Verification items for this drawing (mm, ordinates from the low corner). A direction names the side the tool comes from. Round coordinates to 2 decimals unless told otherwise and drop trailing zeros. Write each loop counter-clockwise with the first axis right and the second up, starting at its lowest first coordinate (ties: lowest second). Pieces come first, ordered by that corner, then holes. Notation, with made-up numbers: (28, 6) -> (58, 6) arc R23 ccw to (58, 37) -> close; hole circle Ø3 at (45.5, -7.75). An arc over 180 degrees is marked (long way). Put each result on its own line as item: value. Start each with the question number.
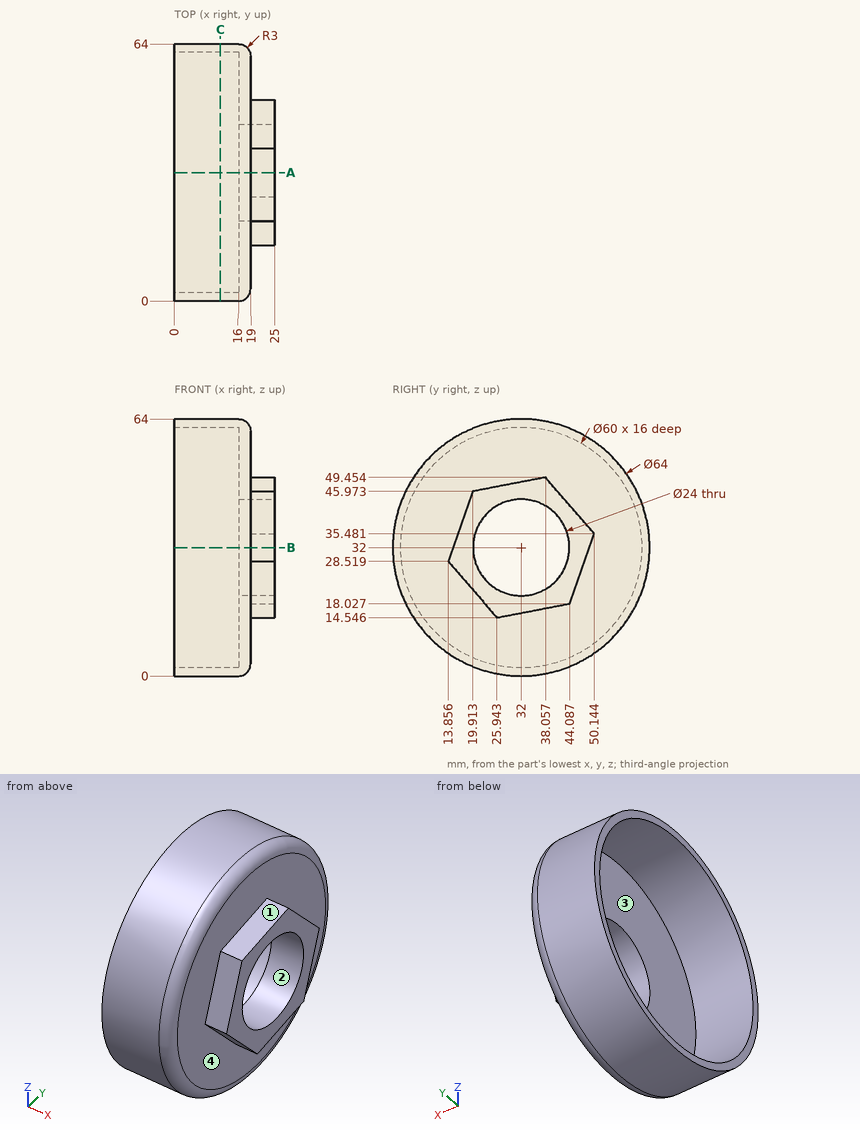
(1) Sectioned sample at B-B (z = 32). Record the cut outline in (x, y).
(2) Sectioned sample at C-C (x = 11.5). Record the cut outline in (y, z).
(3) Go/stop test with flat-tipped pins: pin 1 Ø1 at (y, z) = (39.5, 52.5) entering from +X; pin 2 Ø10 at (x, z) = (19.5, 51) entering from +Y (1 decimal); pin 3 Ø1 at (x, z) = (20.5, 53) entering from +Y (3 decimals); pin 4 Ø4 at (x, y) = (22.5, 14) entering from -Z. Record where each tip stops, or that it passes through.
(4) Material ranges on L1, parallel to Y at x = 7.25, z = 32; L2, parallel to Z at x = 2.75, y = 5 (1 decimal); L3, parallel to Z at x = 11.75, y = 34.5 (1 decimal), recorded low to high. Write a range as from..to.
(5) Sectioned sample at A-A (y = 32). Record the cut outline in (x, z).
(6) Set-up check for the marked faces 1, 2, 3 and 4: record each of +Z, -Z, +X, -X, +Y, -Y from which the full face is reachable in a straight line by a thin tool's end or side.
Found:
1. outline: (0, 0) -> (16, 0) arc R3 ccw to (19, 3) -> (19, 15.06) -> (25, 15.06) -> (25, 20) -> (16, 20) -> (16, 2) -> (0, 2) -> close; (0, 62) -> (16, 62) -> (16, 44) -> (25, 44) -> (25, 48.94) -> (19, 48.94) -> (19, 61) arc R3 ccw to (16, 64) -> (0, 64) -> close
2. outline: circle Ø64 at (32, 32); hole circle Ø60 at (32, 32)
3. pin 1: x = 19
3. pin 2: y = 60.3
3. pin 3: through
3. pin 4: z = 26.04
4. L1: 0..2, 62..64
4. L2: 14.8..18.9, 45.1..49.2
4. L3: 0.1..2.1, 61.9..63.9
5. outline: (0, 0) -> (16, 0) arc R3 ccw to (19, 3) -> (19, 15.71) -> (25, 15.71) -> (25, 20) -> (16, 20) -> (16, 2) -> (0, 2) -> close; (0, 62) -> (16, 62) -> (16, 44) -> (25, 44) -> (25, 48.29) -> (19, 48.29) -> (19, 61) arc R3 ccw to (16, 64) -> (0, 64) -> close
6. face 1: +Z, +X, -Y
6. face 2: +X, -X
6. face 3: -X
6. face 4: +X
